Source: three-view drawing plus pictorial views. Frame: mm from the lowest corner of the part. A direction names the side the tool comes from. Give positions to 0.01 mm unless a question says otherwise; leave off trailing zeros. Loops run counter-clockwise (first coordinate to the right, second up) from the corner with the lowest first, then second, coordinate; pieces in that order, holes last. Notation, with made-up numbers: M 44,7 L 77,7 A23 cw 77,16 Z; hole C 3,13.5 d5. An arc over 180 degrees is marked long. Put each result on its own line as item: value. Start each with the question number.
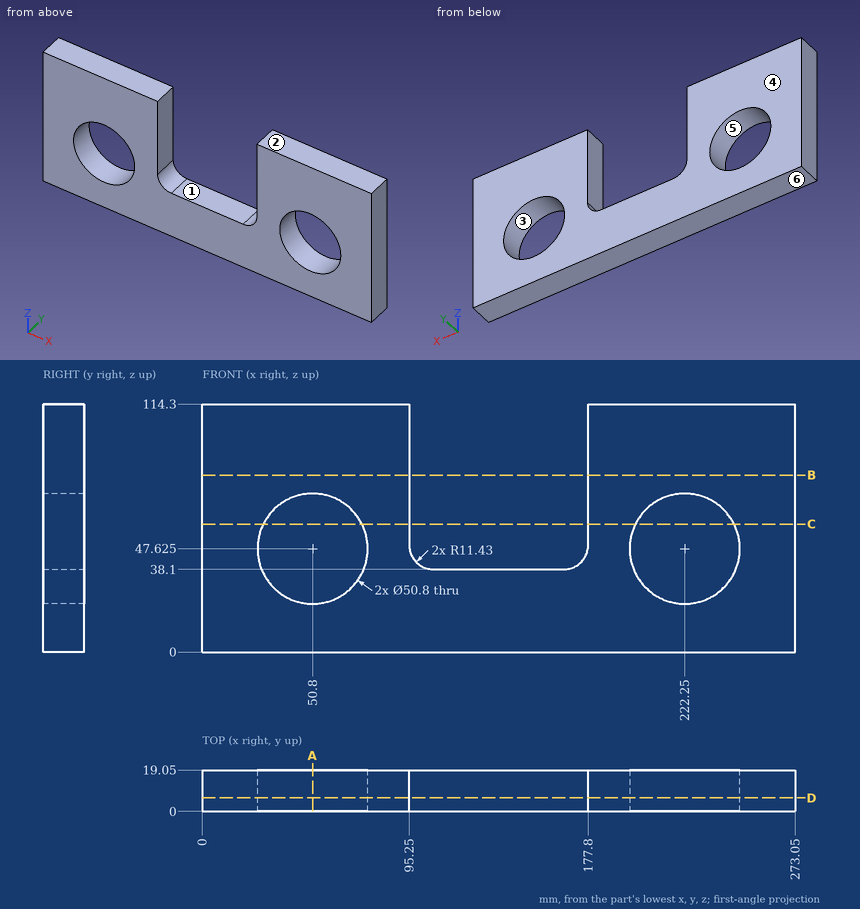
1. Pull-direction query (Z, two-part tool) for the marked faces 3, 4, 5 and 6; classes: released by +Z, released by -Z, zero draft, split by the parting line, or undercut.
2. Section C-C, the plane z = 59. Output: boundary loops of the cut face in (x, y).
3. Ray query, line 1 (X direction, y = 13.5, z = 38); line 2 (X direction, y = 15.5, z = 35); line 3 (X direction, y = 6.75, z = 43). Return the intervals inside material, ascending.
4. Set-up query: the marked faces 1 and 2. Return all of +Z, -Z, +X, -X, +Y, -Y with unobstructed straight access to the full face (end or side cutting, diameter ignored); none if empty.
5. Section B-B, the plane z = 81.5. Output: boundary loops of the cut face in (x, y), plus the area to 3 significant figures.
6. Section A-A, the plane x = 50.8. Output: boundary loops of the cut face in (y, z) (3 decimals).
7. Section D-D, the plane y = 6.25. Output: boundary loops of the cut face in (x, z) (3 decimals), plus the area to 3 significant figures.
8. Contact query for flat-ended pins moving along their axis: pin 1 (5.5 mm diameter, centred on x = 139, y = 9, fed in from +Z); pin 2 (3 mm diameter, centred on x = 170, y = 16, fed in from +Z). Output: stop coordinate, or through.
Results found:
1. face 3: undercut
1. face 4: zero draft
1. face 5: undercut
1. face 6: released by -Z
2. outline: M 0,0 L 28.09,0 L 28.09,19.05 L 0,19.05 Z; M 73.51,0 L 95.25,0 L 95.25,19.05 L 73.51,19.05 Z; M 177.8,0 L 199.54,0 L 199.54,19.05 L 177.8,19.05 Z; M 244.96,0 L 273.05,0 L 273.05,19.05 L 244.96,19.05 Z
3. line 1: 0 to 27.29, 74.31 to 198.74, 245.76 to 273.05
3. line 2: 0 to 28.76, 72.84 to 200.21, 244.29 to 273.05
3. line 3: 0 to 25.82, 75.78 to 97.3, 175.75 to 197.27, 247.23 to 273.05
4. face 1: +Z, +Y, -Y
4. face 2: +Z, +X, -X, +Y, -Y
5. outline: M 0,0 L 95.25,0 L 95.25,19.05 L 0,19.05 Z; M 177.8,0 L 273.05,0 L 273.05,19.05 L 177.8,19.05 Z
5. area: 3,630 mm²
6. outline: M 0,0 L 19.05,0 L 19.05,22.225 L 0,22.225 Z; M 0,73.025 L 19.05,73.025 L 19.05,114.3 L 0,114.3 Z
7. outline: M 0,0 L 273.05,0 L 273.05,114.3 L 177.8,114.3 L 177.8,49.53 A11.43 cw 166.37,38.1 L 106.68,38.1 A11.43 cw 95.25,49.53 L 95.25,114.3 L 0,114.3 Z; hole C 50.8,47.625 d50.8; hole C 222.25,47.625 d50.8
7. area: 20,900 mm²
8. pin 1: z = 38.1
8. pin 2: z = 39.32
